from build123d import *

# Parameters (mm, degrees)
SKETCH1_R           = 14.2875
SKETCH1_R_2         = 2.0193
BOSS_EXTRUDE1_DEPTH = 6.35
SKETCH3_R           = 2.0193
SKETCH3_R_2         = 14.2875
BOSS_EXTRUDE3_DEPTH = 6.35


with BuildPart() as part:
    # Sketch1 → Boss-Extrude1 (new body)
    with BuildSketch(Plane(origin=(0, 0, 0), x_dir=(1, 0, 0), z_dir=(0, 1, 0))):
        with BuildLine():
            Line((-16.51, -19.05), (16.51, -19.05))
            ThreePointArc((16.51, -19.05), (18.306051224, -18.306051224), (19.05, -16.51))
            Line((19.05, -16.51), (19.05, -15.24))
            ThreePointArc((19.05, -15.24), (19.793948776, -13.443948776), (21.59, -12.7))
            Line((21.59, -12.7), (35.56, -12.7))
            ThreePointArc((35.56, -12.7), (37.356051224, -11.956051224), (38.1, -10.16))
            Line((38.1, -10.16), (38.1, 10.16))
            ThreePointArc((38.1, 10.16), (37.356051224, 11.956051224), (35.56, 12.7))
            Line((35.56, 12.7), (21.59, 12.7))
            ThreePointArc((21.59, 12.7), (19.793948776, 13.443948776), (19.05, 15.24))
            Line((19.05, 15.24), (19.05, 16.51))
            ThreePointArc((19.05, 16.51), (18.306051224, 18.306051224), (16.51, 19.05))
            Line((16.51, 19.05), (-16.51, 19.05))
            ThreePointArc((-16.51, 19.05), (-18.306051224, 18.306051224), (-19.05, 16.51))
            Line((-19.05, 16.51), (-19.05, 15.24))
            ThreePointArc((-19.05, 15.24), (-19.793948776, 13.443948776), (-21.59, 12.7))
            Line((-21.59, 12.7), (-35.56, 12.7))
            ThreePointArc((-35.56, 12.7), (-37.356051224, 11.956051224), (-38.1, 10.16))
            Line((-38.1, 10.16), (-38.1, -10.16))
            ThreePointArc((-38.1, -10.16), (-37.356051224, -11.956051224), (-35.56, -12.7))
            Line((-35.56, -12.7), (-21.59, -12.7))
            ThreePointArc((-21.59, -12.7), (-19.793948776, -13.443948776), (-19.05, -15.24))
            Line((-19.05, -15.24), (-19.05, -16.51))
            ThreePointArc((-19.05, -16.51), (-18.306051224, -18.306051224), (-16.51, -19.05))
        make_face()
        Circle(SKETCH1_R, mode=Mode.SUBTRACT)
        with Locations((-31.75, 0)):
            Circle(SKETCH1_R_2, mode=Mode.SUBTRACT)
        with Locations((-19.05, 0)):
            Circle(SKETCH1_R_2, mode=Mode.SUBTRACT)
        with Locations((19.05, 0)):
            Circle(SKETCH1_R_2, mode=Mode.SUBTRACT)
        with Locations((31.75, 0)):
            Circle(SKETCH1_R_2, mode=Mode.SUBTRACT)
    extrude(amount=BOSS_EXTRUDE1_DEPTH)

    # Sketch3 → Boss-Extrude3 (add)
    with BuildSketch(Plane(origin=(0, 6.35, 0), x_dir=(1, 0, 0), z_dir=(0, 1, 0))):
        with BuildLine():
            ThreePointArc((-91.701718319, 75.495704333), (-128.973082608, 63.375659956), (-141.093126985, 26.104295667))
            Line((-141.093126985, 26.104295667), (-35.56, 12.7))
            Line((-35.56, 12.7), (-21.59, 12.7))
            ThreePointArc((-21.59, 12.7), (-19.793948776, 13.443948776), (-19.05, 15.24))
            Line((-19.05, 15.24), (-19.05, 16.51))
            ThreePointArc((-19.05, 16.51), (-18.306051224, 18.306051224), (-16.51, 19.05))
            Line((-16.51, 19.05), (16.51, 19.05))
            ThreePointArc((16.51, 19.05), (18.306051224, 18.306051224), (19.05, 16.51))
            Line((19.05, 16.51), (19.05, 15.24))
            ThreePointArc((19.05, 15.24), (19.793948776, 13.443948776), (21.59, 12.7))
            Line((21.59, 12.7), (35.56, 12.7))
            Line((35.56, 12.7), (-91.701718319, 75.495704333))
        make_face()
        with Locations((-134.357934894, 32.839487758)):
            Circle(SKETCH3_R, mode=Mode.SUBTRACT)
        with Locations((-116.397422652, 50.8)):
            Circle(SKETCH3_R_2, mode=Mode.SUBTRACT)
        with Locations((-98.43691041, 68.760512242)):
            Circle(SKETCH3_R, mode=Mode.SUBTRACT)
    extrude(amount=-BOSS_EXTRUDE3_DEPTH)


solid = part.part
Input: part model. Units: mm. Frame: model coordinates. A direction names the side the tool comes from. Coordinates: 2 decimals unless noted, no trailing zeros. Loops run counter-clockwise (first coordinate to the right, second up) from the corner with the lowest first, then second, coordinate; pieces in that order, holes last. Notation, with made-up numbers: (-11, 48) -> (16, 48) arc R28 ccw to (16, 73) -> close; hole circle Ø10 at (49.25, 7.25). An arc over 180 degrees is marked (long way). One line per item, written item: value.
(1) Pin query (flat end, axial travel): pin 1 Ø1.5 at (y, z) = (4, -28.5) entering from -X; pin 2 Ø1.5 at (x, y) = (-41.5, 3.5) entering from +Z; pin 3 Ø1 at (y, z) = (5.5, -10) entering from -X; pin 4 Ø2.5 at (x, z) = (-19.05, 0) entering from -Y. Return the tip coordinate at first contact, or that it passes through.
Answer below:
pin 1: stops at x = -141.47
pin 2: stops at z = -13.36
pin 3: stops at x = -38.1
pin 4: passes through
(2) Cut plane C-C (y = 2). Give the number of separate pieces and of enclosed holes in the cut face, then the cut area to 3 significant figures.
Answer below:
separate pieces: 1
enclosed holes: 8
area: 6,850 mm2
(3) Ray query, line 1 along X through (y, z) = (2.25, 0); line 2 along X through (y, z) = (1.5, -38); line 3 along X through (y, z) = (2, 15.5). Return the intervals inside material, ascending.
Answer below:
line 1: x = -38.1 to -33.77, -29.73 to -21.07, -17.03 to -14.29, 14.29 to 17.03, 21.07 to 29.73, 33.77 to 38.1
line 2: x = -141.31 to -122.75, -110.05 to -15.71
line 3: x = -19.05 to 19.05
(4) Cut plane D-D (z = -20.5). Output: boundary loops of the cut face in (x, y), then the cut area to 3 significant figures.
Answer below:
outline: (-96.97, 0) -> (19.75, 0) -> (19.75, 6.35) -> (-96.97, 6.35) -> close
area: 741 mm2
(5) Set-up query: faces 4 (the face through (28, 3, 12.7)), 5 (the face through (33.676, 3.131, -0.607)), 6 (the face through (-29, 3, 12.7)). Return all of +Z, -Z, +X, -X, +Y, -Y with unobstructed straight access to the full face (end or side cutting, diameter ignored); none if empty.
Answer below:
face 4: +Z, +X, +Y, -Y
face 5: +Y, -Y
face 6: +Z, -X, +Y, -Y
(6) Draft query along X for faces 1 (the face through (-53, 6.35, -29)), 2 (the face through (-118.257, 3.219, -64.966)), 3 (the face through (-38.1, 3, 0)). Return one class per face: pulls with the +X half, pulls with the -X half, needs draft (parallel to the pull), parting line crosses it, or undercut.
Answer below:
face 1: needs draft
face 2: undercut
face 3: pulls with the -X half
(7) Cut plane B-B (x = -31.75). Output: boundary loops of the cut face in (y, z), then the cut area to 3 significant figures.
Answer below:
outline: (0, -45.91) -> (6.35, -45.91) -> (6.35, -2.02) -> (0, -2.02) -> close; (0, 2.02) -> (6.35, 2.02) -> (6.35, 12.7) -> (0, 12.7) -> close
area: 347 mm2
(8) Cut plane A-A (z = -4.5). Output: boundary loops of the cut face in (x, y), then the cut area to 3 significant figures.
Answer below:
outline: (-38.1, 0) -> (-13.56, 0) -> (-13.56, 6.35) -> (-38.1, 6.35) -> close; (13.56, 0) -> (38.1, 0) -> (38.1, 6.35) -> (13.56, 6.35) -> close
area: 312 mm2
